```python
from build123d import *

# Parameters (mm, degrees)
F0_R      = 25.4
F1_DEPTH  = 3.175
F2_R      = 19.685
F3_DEPTH  = 38.1
F4_R      = 25.4
F5_DEPTH  = 58.42
F7_DEPTH  = 25.401
F10_D     = 9.9314
F12_DEPTH = 25.4
F15_DEPTH = 50.8010001
F16_SIZE  = 0.508
F18_D     = 7.9375


with BuildPart() as f1:
    # F0 (on Right) → F1 (new body)
    with BuildSketch(Plane.YZ):
        Circle(F0_R)
    extrude(amount=F1_DEPTH)

    # F2 (on face) → F3 (join)
    with BuildSketch(Plane.YZ.offset(3.175)):
        Circle(F2_R)
    extrude(amount=-F3_DEPTH)

    # F4 (on Right) → F5 (join)
    with BuildSketch(Plane.YZ):
        Circle(F4_R)
    extrude(amount=F5_DEPTH)

    # F6 (on Front) → F7 (cut, through all)
    with BuildSketch(Plane.XZ):
        Polygon((50.8, 25.4), (3.175, 25.4), (3.175, -25.4), (58.42, -25.4), (58.42, 25.4), align=None)
    extrude(amount=F7_DEPTH, mode=Mode.SUBTRACT)

    # F10 (through all)
    with Locations(Plane.XZ):
        with Locations((29.845, 0)):
            Hole(F10_D / 2)

    # F11 (on Top) → F12 (cut, symmetric)
    with BuildSketch(Plane.XY):
        Polygon((27.3418057965, 3.81), (26.67, 0), (33.02, 0), (32.3481942035, 3.81), align=None)
    extrude(amount=F12_DEPTH, both=True, mode=Mode.SUBTRACT)

    # F14 (on offset) → F15 (cut, through all)
    with BuildSketch(Plane.XZ.offset(25.4)):
        with BuildLine():
            ThreePointArc((29.845, 25.431730181), (55.276730181, 0), (29.845, -25.431730181))
            Line((29.845, -25.431730181), (29.845, -32.23392232))
            Line((29.845, -32.23392232), (58.42, -32.23392232))
            Line((58.42, -32.23392232), (58.42, 32.23392232))
            Line((58.42, 32.23392232), (29.845, 32.23392232))
            Line((29.845, 32.23392232), (29.845, 25.431730181))
        make_face()
    extrude(amount=-F15_DEPTH, mode=Mode.SUBTRACT)

    # F16
    f16_edges = [f1.edges().sort_by_distance(p)[0] for p in [
        (26.67, 0, -14.609028),
        (26.67, 0, 14.609028),
        (33.02, 0, -14.525409),
        (33.02, 0, 14.525409),
    ]]
    chamfer(f16_edges, length=F16_SIZE)

    # F18 (through all)
    with Locations(Plane.XZ.offset(25.4)):
        with Locations((-19.05, 0)):
            Hole(F18_D / 2)


solid = f1.part
```
Could you check a few things on this model? Use its own coordinates, in mm. A direction names the side the tool comes from. Round coordinates to 2 decimals unless told otherwise and drop trailing zeros. Loops run counter-clockwise (first coordinate to the right, second up) from the corner with the lowest first, then second, coordinate; pieces in that order, holes last. Notation, with made-up numbers: (79.25, -33) - (104.25, -33) arc R14 cw to (104.25, -18) - close; hole circle Ø11 at (64, 17). An arc over 180 degrees is marked (long way). Use CSV: the item, a comma, the result in double quotes.
Item 1: If we section it at B-B on y = 14.5: Count the separate pieces of the cut face and the enclosed holes in it, then the cut area to 3 significant figures.
Here are the results:
separate pieces,"1"
enclosed holes,"2"
area,"2,970 mm²"
Item 2: If we section it at A-A on z = 0: List the corners of the cut face in (x, y) for me (3 decimals), then the cut area to 3 significant figures.
Here are the results:
outline,"(-34.925, -19.685) - (-23.019, -19.685) - (-23.019, 19.685) - (-34.925, 19.685) - close; (-15.081, -19.685) - (0, -19.685) - (0, -25.4) - (3.175, -25.4) - (3.175, 0) - (24.879, 0) - (24.879, 25.4) - (0, 25.4) - (0, 19.685) - (-15.081, 19.685) - close; (34.811, 0) - (55.277, 0) - (55.277, 25.4) - (34.811, 25.4) - close"
area,"2,290 mm²"
Item 3: If we mould it in two halves opening along X, with no side actions, what happens to faces 1 (the flat face through (15, 0, 0)), 2 (the cylindrical face through (-15.085, 0.276, 0.174)), 3 (the flat face through (3.175, -10, 0))? For each: pulls with the +X half, pulls with the -X half, needs draft (parallel to the pull), parting line crosses it, or undercut.
Here are the results:
face 1,"needs draft"
face 2,"undercut"
face 3,"pulls with the +X half"
Item 4: For faces 4 (the cylindrical face through (-17.2, 18.2, -7.5)), 5 (the flat face through (32.644, 2.132, -14.437)), 6 (the flat face through (42, 0, 0)), 7 (the cylindrical face through (21.11, 24.227, 7.629)), which set-ups out of +Z, -Z, +X, -X, +Y, -Y let a thin tool reach every point of the face, with its end or its side?
Here are the results:
face 4,"-X"
face 5,"+Z, -Z, -Y"
face 6,"+Z, -Z, +X, -Y"
face 7,"+X, -X"
Item 5: If we section it at D-D on x = -19.05: List the corners of the cut face in (y, z) for me (3 decimals), then the cut area to 3 significant figures.
Here are the results:
outline,"(-19.281, -3.969) arc R19.685 ccw to (19.281, -3.969) - close; (-19.281, 3.969) - (19.281, 3.969) arc R19.685 ccw to start"
area,"907 mm²"
Item 6: Will these pins go through, and if not, where does the flat tip stop? pin 1 (5 mm diameter, centred on y = 16.5, z = 3.5, fed in from +X); pin 2 (12 mm diameter, centred on x = -24.5, y = 4.5, fed in from +Z) (3 decimals); pin 3 (7.5 mm diameter, centred on y = -11.5, z = 0, fed in from +X) (3 decimals).
Here are the results:
pin 1,"stops at x = 55.26"
pin 2,"stops at z = 19.685"
pin 3,"stops at x = 3.175"
Item 7: I need wall thicknesses on L1, parallel to X at y = 3, z = 0 (3 decimals); L2, parallel to X at y = -5, z = 0 (3 decimals); L3, parallel to X at y = -21, z = -2.5 (3 decimals). Which ranges of each line are inside material? Lowest first, please. Write a range as [from, to].
Here are the results:
L1,"x = [-34.925, -23.019], [-15.081, 24.879], [34.811, 55.277]"
L2,"x = [-34.925, -23.019], [-15.081, 3.175]"
L3,"x = [0, 3.175]"
